Geometry: final body of the model. Coordinates: model frame, mm. Give positions to 0.01 mm unless a question says otherwise; leave off trailing zeros. Use a Markdown table: item, result. Add a question column.
1) Pin query (flat end, axial travel): pin 1 (4 mm diameter, centred on x = -110, z = -75, fed in from -Y); pin 2 (0.9 mm diameter, centred on y = -1, z = -102.5, fed in from -X); pin 3 (0.9 mm diameter, centred on y = -1, z = -102.5, fed in from +X). Return the tip coordinate at first contact, or that it passes through.
2) Draft query along X for faces 1 (the flat face through (-2, -3, 1)), 2 (the cylindrical face through (-75.747, -1.521, -39.879)). Return one class per face: +X half, -X half, draft (parallel to the pull), parting line (faces both ways), or undercut.
3) Line query: line 1 (Z direction, x = -30, y = -0.55); line 2 (Z direction, x = -44.5, y = -0.45). Output: solid intervals per line, ascending.
```python
from build123d import *

# Parameters (mm, degrees)
F1_DEPTH = 3
F2_R     = 2.75
F3_DEPTH = 3
F4_R     = 2.5
F5_DEPTH = 3
F6_R     = 2.5
F7_DEPTH = 3
F8_R     = 4.99999


# Not quite as in the source:
# - a fillet or chamfer is up to 0.001 mm smaller than in the source, because OpenCascade refuses the exact size


with BuildPart() as f1:
    # F0 (on Front) → F1 (new body)
    with BuildSketch(Plane.XZ):
        Polygon((140, -105), (145, -105), (145, 105), (-145, 105), (-145, -105), (-140, -105), (-140, -95), (-134.5, -95), (-134.5, -105), (134.5, -105), (134.5, -95), (140, -95), align=None)
    extrude(amount=F1_DEPTH)

    # F2 (on face) → F3 (cut, through all)
    with BuildSketch(Plane.XZ.offset(3)):
        with Locations((-110, 100)):
            Circle(F2_R)
        with Locations((-138, -40)):
            Circle(F2_R)
        with Locations((-45, 100)):
            Circle(F2_R)
        with Locations((-73, -40)):
            Circle(F2_R)
    extrude(amount=-F3_DEPTH, mode=Mode.SUBTRACT)

    # F4 (on face) → F5 (cut, through all)
    with BuildSketch(Plane.XZ.offset(3)):
        with Locations((-30, 100)):
            Circle(F4_R)
        with Locations((140, 100)):
            Circle(F4_R)
        with Locations((75, -85)):
            Circle(F4_R)
        with Locations((-30, -40)):
            Circle(F4_R)
    extrude(amount=-F5_DEPTH, mode=Mode.SUBTRACT)

    # F6 (on face) → F7 (cut, through all)
    with BuildSketch(Plane.XZ.offset(3)):
        with Locations((-110, -75)):
            Circle(F6_R)
        with Locations((-42.5, -75)):
            Circle(F6_R)
    extrude(amount=-F7_DEPTH, mode=Mode.SUBTRACT)

    # F8 (radius 5 in the source; OpenCascade refuses exactly that, so slightly less here)
    f8_edges = [f1.edges().sort_by_distance(p)[0] for p in [
        (-145, -1.5, 105),
        (145, -1.5, 105),
        (145, -1.5, -105),
        (-145, -1.5, -105),
    ]]
    fillet(f8_edges, radius=F8_R)


solid = f1.part
```
Found:
| question | item | result |
|---|---|---|
| 1 | pin 1 | through |
| 1 | pin 2 | x = -144.56 |
| 1 | pin 3 | x = 144.56 |
| 2 | face 1 | draft |
| 2 | face 2 | undercut |
| 3 | line 1 | -105 to -42.5, -37.5 to 97.5, 102.5 to 105 |
| 3 | line 2 | -105 to -76.5, -73.5 to 97.3, 102.7 to 105 |
